Geometry check sheet. Reference: drawing and pictorial views, mm from the part's lowest x, y, z. Give positions to 0.01 mm unless a question says otherwise; leave off trailing zeros. Write each loop counter-clockwise with the first axis right and the second up, starting at its lowest first coordinate (ties: lowest second). Pieces come first, ordered by that corner, then holes. Notation, with made-up numbers: M 31.25,60 L 43.25,60 A27 cw 43.25,88 Z; hole C 24.25,66.25 d7. An arc over 180 degrees is marked long. Write item = value, one per line. Start each with the question number.
1) Cross-section at A-A, the plane z = 3.75. Record the cut outline in (x, y).
2) Scan lines: line 1 along X through (y, z) = (2.75, 3.75); line 2 along Y through (x, z) = (23, 1.5); line 3 along Y through (x, z) = (11, 3.5). Record each from-to range of solid material in increasing order. Write a range as [from, to].
3) Cross-section at B-B, the plane y = 3.75. Record the cut outline in (x, z), plus the area to 3 significant figures.
4) Cross-section at C-C, the plane x = 31.5. Record the cut outline in (y, z), plus the area to 3 significant figures.
5) Go/stop test with flat-tipped pins: pin 1 (3 mm diameter, centred on x = 21, y = 2, fed in from -Z); pin 2 (1 mm diameter, centred on x = 10.5, z = 5.5, fed in from -Y) (1 decimal); pin 3 (2 mm diameter, centred on x = 37.5, y = 2.5, fed in from +Z). Record where each tip stops, or that it passes through.
6) Mould release check, pull along X, two halves, no side actions. Record for the marked faces 1, 2 and 3: released by +X, released by -X, zero draft, split by the parting line, or undercut.
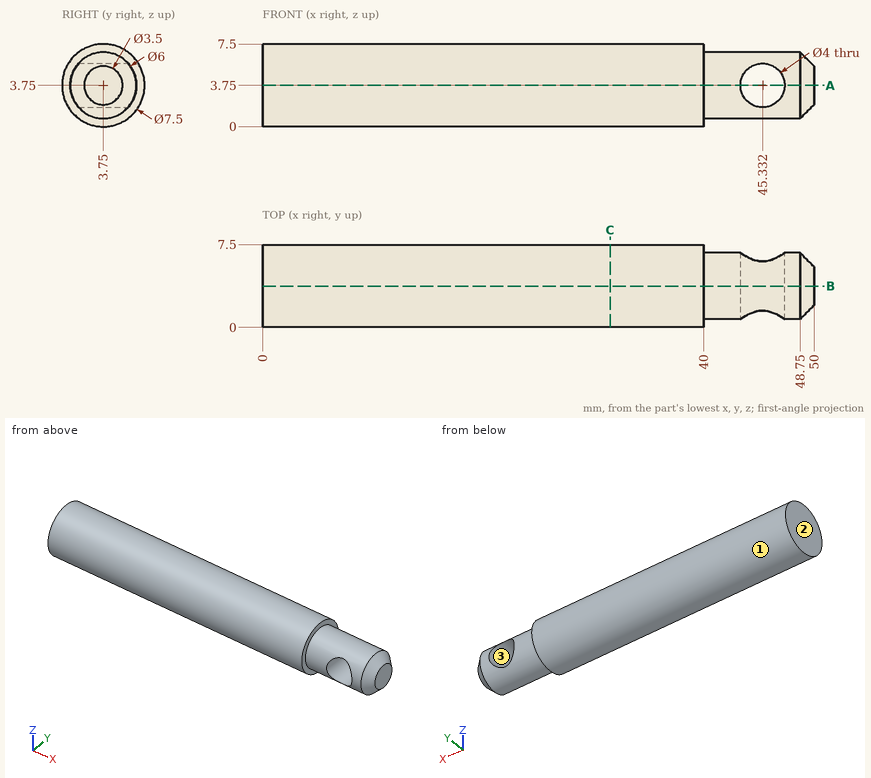
Reply:
q1.outline = M 0,0 L 40,0 L 40,0.75 L 43.33,0.75 L 43.33,6.75 L 40,6.75 L 40,7.5 L 0,7.5 Z; M 47.33,0.75 L 48.75,0.75 L 50,2 L 50,5.5 L 48.75,6.75 L 47.33,6.75 Z
q2.line_1 = [0, 43.33], [47.33, 50]
q2.line_2 = [0.75, 6.75]
q2.line_3 = [0.01, 7.49]
q3.outline = M 0,0 L 40,0 L 40,0.75 L 48.75,0.75 L 50,2 L 50,5.5 L 48.75,6.75 L 40,6.75 L 40,7.5 L 0,7.5 Z; hole C 45.33,3.75 d4
q3.area = 346 mm2
q4.outline = C 3.75,3.75 d7.5
q4.area = 44.2 mm2
q5.pin_1 = 0.01
q5.pin_2 = 0.2
q5.pin_3 = 7.49
q6.face_1 = zero draft
q6.face_2 = released by -X
q6.face_3 = undercut
